Verification items for the finished model (mm, model axes). A direction names the side the tool comes from. Coordinates: 2 decimals unless noted, no trailing zeros. Write each loop counter-clockwise with the first axis right and the second up, starting at its lowest first coordinate (ties: lowest second). Pieces come first, ordered by that corner, then holes. Notation, with made-up numbers: (-34.5, -9.75) -> (-20.5, -9.75) arc R19 cw to (-20.5, -3.75) -> close; hole circle Ø4 at (-36, 50.25). An arc over 180 degrees is marked (long way). Answer in a Markdown table with one row per item.
```python
from build123d import *

# Parameters (mm, degrees)
SKETCH1_R           = 5.5
BOSS_EXTRUDE1_DEPTH = 7
SKETCH2_R           = 1.25
CUT_EXTRUDE1_DEPTH  = 12
SKETCH3_R           = 1.25
CUT_EXTRUDE2_DEPTH  = 12
BOSS_EXTRUDE3_DEPTH = 7
FILLET1_R           = 3
SKETCH5_R           = 1
CUT_EXTRUDE3_DEPTH  = 7
SKETCH6_R           = 3
SKETCH6_W           = 6
SKETCH6_H           = 6
BOSS_EXTRUDE5_DEPTH = 12
SKETCH8_R           = 1.25
CUT_EXTRUDE4_DEPTH  = 10
SKETCH9_R           = 2
CUT_EXTRUDE5_DEPTH  = 24
SKETCH10_W          = 5
SKETCH10_H          = 6
CUT_EXTRUDE6_DEPTH  = 4
SKETCH12_R          = 6.5
CUT_EXTRUDE9_DEPTH  = 4
SKETCH13_W          = 35
SKETCH13_H          = 0.258068079
CUT_EXTRUDE10_DEPTH = 11
SKETCH14_W          = 33.43687833
SKETCH14_H          = 0.407122994
CUT_EXTRUDE11_DEPTH = 11
SKETCH15_R          = 1
BOSS_EXTRUDE6_DEPTH = 2
SKETCH16_R          = 1.25
CUT_EXTRUDE12_DEPTH = 5


with BuildPart() as part:
    # Sketch1 → Boss-Extrude1 (new body)
    with BuildSketch(Plane.XY):
        Polygon((0, 0), (0, 35), (32, 35), (35, 8), (35, 0), align=None)
        with Locations((14.5, 17.5)):
            Circle(SKETCH1_R, mode=Mode.SUBTRACT)
    extrude(amount=BOSS_EXTRUDE1_DEPTH)

    # Sketch2 → Cut-Extrude1 (cut)
    with BuildSketch(Plane.XZ):
        with Locations((6, 3.5)):
            Circle(SKETCH2_R)
    extrude(amount=-CUT_EXTRUDE1_DEPTH, mode=Mode.SUBTRACT)

    # Sketch3 → Cut-Extrude2 (cut)
    with BuildSketch(Plane.XZ):
        with Locations((24, 3.5)):
            Circle(SKETCH3_R)
    extrude(amount=-CUT_EXTRUDE2_DEPTH, mode=Mode.SUBTRACT)

    # Sketch4 → Boss-Extrude3 (add)
    with BuildSketch(Plane.XY.offset(7)):
        Polygon((16.95692267, 41), (16.95692267, 35), (24.95692267, 35), (22.287605299, 41), align=None)
    extrude(amount=-BOSS_EXTRUDE3_DEPTH)

    # Fillet1
    fillet1_edges = [part.edges().sort_by_distance(p)[0] for p in [
        (22.287605299, 41, 3.5),
        (16.95692267, 41, 3.5),
    ]]
    fillet(fillet1_edges, radius=FILLET1_R)

    # Sketch5 → Cut-Extrude3 (cut)
    with BuildSketch(Plane.XY.offset(7)):
        with Locations((19.95692267, 38)):
            Circle(SKETCH5_R)
    extrude(amount=-CUT_EXTRUDE3_DEPTH, mode=Mode.SUBTRACT)

    # Sketch6 → Boss-Extrude5 (add)
    with BuildSketch(Plane(origin=(0, 18, 0), x_dir=(1, 0, 0), z_dir=(0, 1, 0))):
        with Locations((4.401568824, -10)):
            Circle(SKETCH6_R)
        with Locations((24.018340299, -10)):
            Circle(SKETCH6_R)
        with Locations((4.401568824, -7)):
            Rectangle(SKETCH6_W, SKETCH6_H)
        with Locations((24.018340299, -7)):
            Rectangle(SKETCH6_W, SKETCH6_H)
    extrude(amount=BOSS_EXTRUDE5_DEPTH)

    # Sketch8 → Cut-Extrude4 (cut)
    with BuildSketch(Plane(origin=(0, 30, 0), x_dir=(1, 0, 0), z_dir=(0, 1, 0))):
        with Locations(Location((4.401568824, -10, 0), (0, 0, 180))):
            Circle(SKETCH8_R)
        with Locations(Location((24.018340299, -10, 0), (0, 0, 180))):
            Circle(SKETCH8_R)
    extrude(amount=-CUT_EXTRUDE4_DEPTH, mode=Mode.SUBTRACT)

    # Sketch9 → Cut-Extrude5 (cut)
    with BuildSketch(Plane(origin=(0, 35, 0), x_dir=(1, 0, 0), z_dir=(0, 1, 0))):
        with Locations(Location((28.478461335, -3.5, 0), (0, 0, 180))):
            Circle(SKETCH9_R)
    extrude(amount=-CUT_EXTRUDE5_DEPTH, mode=Mode.SUBTRACT)

    # Sketch10 → Cut-Extrude6 (cut)
    with BuildSketch(Plane(origin=(0, 0, 0), x_dir=(-1, 0, 0), z_dir=(0, 0, -1))):
        with Locations((-28.609401926, 18)):
            Rectangle(SKETCH10_W, SKETCH10_H)
    extrude(amount=-CUT_EXTRUDE6_DEPTH, mode=Mode.SUBTRACT)

    # Sketch12 → Cut-Extrude9 (cut)
    with BuildSketch(Plane(origin=(0, 0, 0), x_dir=(-1, 0, 0), z_dir=(0, 0, -1))):
        with Locations((-14.5, 17.5)):
            Circle(SKETCH12_R)
    extrude(amount=-CUT_EXTRUDE9_DEPTH, mode=Mode.SUBTRACT)

    # Sketch13 → Cut-Extrude10 (cut)
    with BuildSketch(Plane(origin=(0, 41, 0), x_dir=(1, 0, 0), z_dir=(0, 1, 0))):
        with Locations((17.5, -6.870965961)):
            Rectangle(SKETCH13_W, SKETCH13_H)
    extrude(amount=-CUT_EXTRUDE10_DEPTH, mode=Mode.SUBTRACT)

    # Sketch14 → Cut-Extrude11 (cut)
    with BuildSketch(Plane(origin=(0, 41, 0), x_dir=(1, 0, 0), z_dir=(0, 1, 0))):
        with Locations((16.718439165, -6.538370424)):
            Rectangle(SKETCH14_W, SKETCH14_H)
    extrude(amount=-CUT_EXTRUDE11_DEPTH, mode=Mode.SUBTRACT)

    # Sketch15 → Boss-Extrude6 (add)
    with BuildSketch(Plane.XY.offset(6.334808927)):
        with Locations((19.95692267, 38)):
            Circle(SKETCH15_R)
    extrude(amount=-BOSS_EXTRUDE6_DEPTH)

    # Sketch16 → Cut-Extrude12 (cut)
    with BuildSketch(Plane(origin=(0, 0, 0), x_dir=(-1, 0, 0), z_dir=(0, 0, -1))):
        with Locations((-29.943004203, 5.499566532)):
            Circle(SKETCH16_R)
    extrude(amount=-CUT_EXTRUDE12_DEPTH, mode=Mode.SUBTRACT)


solid = part.part
```
1. Access from +Z, -Z, +X, -X, +Y, -Y to the whole of each face (thin tool, end or side, straight path). Record for faces 4 (the face through (8, 35, 3)), 5 (the face through (29, 15, 1)), 6 (the face through (1.402, 24, 9)), 7 (the face through (7.402, 24, 9)), 8 (the face through (5.01, 5.92, 2.74)).
Findings below:
| item | result |
|---|---|
| face 4 | +Z, -Z, -X, +Y |
| face 5 | -Z |
| face 6 | +Z, -X, +Y, -Y |
| face 7 | +Z, +Y, -Y |
| face 8 | -Y |
2. Sectioned sample at B-B, the plane x = 14.5. Record the cut outline in (y, z), and give its area (3 significant figures).
Findings below:
| item | result |
|---|---|
| outline | (0, 0) -> (11, 0) -> (11, 4) -> (12, 4) -> (12, 7) -> (0, 7) -> close; (23, 4) -> (24, 4) -> (24, 0) -> (35, 0) -> (35, 6.33) -> (30, 6.33) -> (30, 7) -> (23, 7) -> close |
| area | 157 mm² |
3. Go/stop test with flat-tipped pins: pin 1 (3 mm diameter, centred on x = 28.48, z = 3.5, fed in from +Y); pin 2 (3 mm diameter, centred on y = 17, z = 2.5, fed in from +X); pin 3 (1.5 mm diameter, centred on y = 21.5, z = 8.5, fed in from +X). Record where each tip stops, or that it passes through.
Findings below:
| item | result |
|---|---|
| pin 1 | stops at y = 11 |
| pin 2 | stops at x = 34.17 |
| pin 3 | stops at x = 27.02 |
4. Sectioned sample at D-D, the plane z = 3.5. Count the separate pieces of the cut face and the enclosed holes in it, and give its area (3 significant figures).
Findings below:
| item | result |
|---|---|
| separate pieces | 1 |
| enclosed holes | 3 |
| area | 919 mm² |
5. Sectioned sample at A-A, the plane z = 7.75. Record the cut outline in (x, y).
Findings below:
| item | result |
|---|---|
| outline | (1.4, 18) -> (7.4, 18) -> (7.4, 30) -> (1.4, 30) -> close; (21.02, 18) -> (27.02, 18) -> (27.02, 30) -> (21.02, 30) -> close |
6. Release check for a two-part mould opening along Y. For faces 1 (the face through (20, 38, 4.335)), 2 (the face through (3.73, 25.07, 11.054)), 3 (the face through (16, 30, 6.7)) record: released by +Y, released by -Y, zero draft, split by the parting line, or undercut.
Findings below:
| item | result |
|---|---|
| face 1 | undercut |
| face 2 | zero draft |
| face 3 | released by +Y |
7. Material ranges on probe 1 along X at (y, z) = (17.5, 4.75); probe 2 along X at (y, z) = (21, 7.25); probe 3 along Z at (x, y) = (24, 26.5), recorded low to high. Write a range as from..to.
Findings below:
| item | result |
|---|---|
| probe 1 | x = 0..9, 20..26.92, 30.04..33.94 |
| probe 2 | x = 1.4..7.4, 21.02..27.02 |
| probe 3 | z = 0..8.75, 11.25..13 |
8. Sectioned sample at C-C, the plane y = 34. Record the cut outline in (x, z), and give its area (3 significant figures).
Findings below:
| item | result |
|---|---|
| outline | (0, 0) -> (32.11, 0) -> (32.11, 6.33) -> (0, 6.33) -> close; hole circle Ø4 at (28.48, 3.5) |
| area | 191 mm² |
